from build123d import *

# Parameters (mm, degrees)
BOSS_EXTRUDE2_DEPTH = 9
BOSS_EXTRUDE3_DEPTH = 19
CHAMFER1_SIZE       = 2
CUT_EXTRUDE1_DEPTH  = 50
SKETCH6_R           = 4.5
CUT_EXTRUDE2_DEPTH  = 50
CUT_EXTRUDE3_DEPTH  = 4
FILLET1_R           = 2


with BuildPart() as part:
    # Sketch1 → Boss-Extrude2 (new, symmetric)
    with BuildSketch(Plane(origin=(0, 0, 0), x_dir=(1, 0, 0), z_dir=(0, 1, 0))):
        with BuildLine():
            Line((-17, -61), (17, -61))
            Line((17, -61), (29, -46))
            Line((29, -46), (44.77708764, -46))
            Line((44.77708764, -46), (44.77708764, 4))
            Line((44.77708764, 4), (35.77708764, 4))
            ThreePointArc((35.77708764, 4), (0, -36), (-35.77708764, 4))
            Line((-35.77708764, 4), (-44.77708764, 4))
            Line((-44.77708764, 4), (-44.77708764, -46))
            Line((-44.77708764, -46), (-29, -46))
            Line((-29, -46), (-17, -61))
        make_face()
    extrude(amount=BOSS_EXTRUDE2_DEPTH, both=True)

    # Sketch3 → Boss-Extrude3 (add, symmetric)
    with BuildSketch(Plane(origin=(0, 0, 0), x_dir=(1, 0, 0), z_dir=(0, 1, 0))):
        with BuildLine():
            Line((36, 0), (33, 0))
            ThreePointArc((33, 0), (0, -33), (-33, 0))
            Line((-33, 0), (-36, 0))
            ThreePointArc((-36, 0), (0, -36), (36, 0))
        make_face()
    extrude(amount=BOSS_EXTRUDE3_DEPTH, both=True)

    # Chamfer1
    chamfer1_edges = [part.edges().sort_by_distance(p)[0] for p in [
        (0, -19, 33),
        (0, 19, 33),
    ]]
    chamfer(chamfer1_edges, length=CHAMFER1_SIZE)

    # Sketch5 → Cut-Extrude1 (cut)
    with BuildSketch(Plane(origin=(0, 0, -4), x_dir=(-1, 0, 0), z_dir=(0, 0, -1))):
        with BuildLine():
            ThreePointArc((-44.77708764, -4.1e-08), (-42.141048685, 6.363961016), (-35.77708764, 9))
            Line((-35.77708764, 9), (-44.77708764, 9))
            Line((-44.77708764, 9), (-44.77708764, -4.1e-08))
        make_face()
        with BuildLine():
            ThreePointArc((-35.77708764, -9), (-42.141048656, -6.363961045), (-44.77708764, -4.1e-08))
            Line((-44.77708764, -4.1e-08), (-44.77708764, -9))
            Line((-44.77708764, -9), (-35.77708764, -9))
        make_face()
    cut_extrude1 = extrude(amount=-CUT_EXTRUDE1_DEPTH, mode=Mode.SUBTRACT)

    # Sketch6 → Cut-Extrude2 (cut)
    with BuildSketch(Plane(origin=(0, 0, -4), x_dir=(-1, 0, 0), z_dir=(0, 0, -1))):
        with Locations((-35.77708764, 0)):
            Circle(SKETCH6_R)
    cut_extrude2 = extrude(amount=-CUT_EXTRUDE2_DEPTH, mode=Mode.SUBTRACT)

    # Sketch7 → Cut-Extrude3 (cut)
    with BuildSketch(Plane(origin=(0, 0, -4), x_dir=(-1, 0, 0), z_dir=(0, 0, -1))):
        with BuildLine():
            Line((-35.77708764, 6), (-35.77708764, 4.5))
            ThreePointArc((-35.77708764, 4.5), (-40.27708764, 0), (-35.77708764, -4.5))
            Line((-35.77708764, -4.5), (-35.77708764, -6))
            ThreePointArc((-35.77708764, -6), (-41.77708764, 0), (-35.77708764, 6))
        make_face()
    cut_extrude3 = extrude(amount=-CUT_EXTRUDE3_DEPTH, mode=Mode.SUBTRACT)

    # Mirror2: Cut-Extrude1, Cut-Extrude2, Cut-Extrude3 across plane
    add(cut_extrude1.mirror(Plane(origin=(0, 0, 0), x_dir=(0, 0, 1), z_dir=(1, 0, 0))), mode=Mode.SUBTRACT)
    add(cut_extrude2.mirror(Plane(origin=(0, 0, 0), x_dir=(0, 0, 1), z_dir=(1, 0, 0))), mode=Mode.SUBTRACT)
    add(cut_extrude3.mirror(Plane(origin=(0, 0, 0), x_dir=(0, 0, 1), z_dir=(1, 0, 0))), mode=Mode.SUBTRACT)

    # Fillet1
    # the kernel refuses this fillet: 2 mm, written as the material it adds along each edge
    with BuildSketch(Plane(origin=(0, -9, 0), x_dir=(0.9996152524995429, 0, -0.027737104576279894), z_dir=(-0.027737104576279894, 0, -0.9996152524995429))) as fillet1_piece_1_section:
        with BuildLine():
            CenterArc((36 + FILLET1_R, FILLET1_R), FILLET1_R, 180, 90)
            Line((36, FILLET1_R), (36, 0))
            Line((36, 0), (36 + FILLET1_R, 0))
        make_face()
    fillet1_piece_1 = revolve(axis=Axis((0, -9, 0), (0, -1, 0)), revolution_arc=183.178845751, mode=Mode.PRIVATE)
    fillet1_piece_1 = split(fillet1_piece_1, bisect_by=Plane(origin=(0, -9, 0), z_dir=(0, 0, 1)), keep=Keep.TOP, mode=Mode.PRIVATE)
    add(fillet1_piece_1)
    with BuildSketch(Plane(origin=(0, 9, 0), x_dir=(0.9996152524995429, 0, -0.027737104576279894), z_dir=(-0.027737104576279894, 0, -0.9996152524995429))) as fillet1_piece_2_section:
        with BuildLine():
            CenterArc((36 + FILLET1_R, -FILLET1_R), FILLET1_R, 90, 90)
            Line((36, -FILLET1_R), (36, 0))
            Line((36, 0), (36 + FILLET1_R, 0))
        make_face()
    fillet1_piece_2 = revolve(axis=Axis((0, 9, 0), (0, -1, 0)), revolution_arc=183.178845751, mode=Mode.PRIVATE)
    fillet1_piece_2 = split(fillet1_piece_2, bisect_by=Plane(origin=(0, 9, 0), z_dir=(0, 0, 1)), keep=Keep.TOP, mode=Mode.PRIVATE)
    add(fillet1_piece_2)


solid = part.part
The model under review builds one solid part; all positions refer to its coordinate system, in mm. A direction names the side the tool comes from. Give positions to 0.01 mm unless a question says otherwise; leave off trailing zeros. Write each loop counter-clockwise with the first axis right and the second up, starting at its lowest first coordinate (ties: lowest second). Pieces come first, ordered by that corner, then holes.
1. Wall thickness on L1, parallel to X at y = 1, z = 44.5; L2, parallel to Y at x = 5, z = 57; L3, parallel to Z at x = -38, y = 7: over which ranges is each line inside the solid? List them lowest first.
2. Tool access review of faces 4 (the flat face through (40, -2, 46)), 5 (the cylindrical face through (-0.79, 15.06, 35.99)), 6 (the cylindrical face through (41.776, -0.132, -2.028)): name each direction out of +Z, -Z, +X, -X, +Y, -Y from which nothing blocks a thin tool from reaching the whole face with its end or side.
3. Draft analysis for pull direction Z (two halves, no side actions). For faces 1 (the cylindrical face through (-0.79, -14.94, 35.99)), 2 (the conical face through (0.73, -17.32, 33.31)), 3 (the cylindrical face through (-35.946, -7.477, -1.975)), state which applies: +Z half, -Z half, draft (parallel to the pull), parting line (faces both ways), or undercut.
4. Add section A-A, the plane x = 0. Write out the cut boundary in (y, z), plus the area to 3 significant figures.
5. For P1, Ø11.5, axis at x = 35.78, y = 0, coming from the +Z side; P2, Ø3, axis at x = 35.5, y = -1.5, coming from the -Z side; P3, Ø3, axis at x = -16.5, y = 10.5, coming from the -Z side; P4, Ø1.1, axis at x = 37.5, z = 8.5, coming from the -Y side, all flat-tipped, find the tip position at first contact; note any pin that passes through.
6. Add section C-C, the plane z = 28. Count the separate pieces of the cut face and the enclosed holes in it, plus the area to 3 significant figures.
7. Add section B-B, the plane z = 53.5. Write out the cut boundary in (x, y).
Worked answers:
1. L1: x = -44.72 to -40.16, -31.39 to 31.39, 40.16 to 44.72
1. L2: y = -9 to 9
1. L3: z = -4 to 46
2. face 4: +Z, +X, +Y, -Y
2. face 5: +Z, +Y
2. face 6: -Z
3. face 1: +Z half
3. face 2: -Z half
3. face 3: undercut
4. outline: (-19, 35) - (-17, 33) - (17, 33) - (19, 35) - (19, 36) - (11, 36) arc R2 cw to (9, 38) - (9, 61) - (-9, 61) - (-9, 38) arc R2 cw to (-11, 36) - (-19, 36) - close
4. area: 562 mm2
5. P1: stops at z = 46
5. P2: passes through
5. P3: stops at z = 27.66
5. P4: stops at y = -9
6. separate pieces: 2
6. enclosed holes: 2
6. area: 984 mm2
7. outline: (-23, -9) - (23, -9) - (23, 9) - (-23, 9) - close
